Study the drawing (mm; zero at the part's minimum x, y, z) and answer. Round coordinates to 2 decimals unless told otherwise and drop trailing zeros. Loops run counter-clockwise (first coordinate to the right, second up) from the corner with the lowest first, then second, coordinate; pieces in that order, holes last. Notation, with made-up numbers: M -31,20.5 L 9,20.5 A27 cw 9,52.5 Z; hole C 6,46.25 d10. An arc over 180 degrees is marked long. Put each result on its own line as item: value. Start each with the question number.
(1) Straight lines are drawn through the part: line 1 (Z direction, x = 50, y = 5); line 2 (X direction, y = 3.75, z = 120.5). For each, find the intervals that lie inside material, in ascending order.
(2) Section C-C, the plane y = 2 is taken. Determine the outline of the cut face in (x, z).
(3) Section A-A, the plane z = 20 is taken. Determine the outline of the cut face in (x, y), then the cut area to 3 significant figures.
(4) Section D-D, the plane z = 114.5 is taken. Determine the outline of the cut face in (x, y).
(5) Section B-B, the plane x = 50 is taken. Determine the outline of the cut face in (y, z).
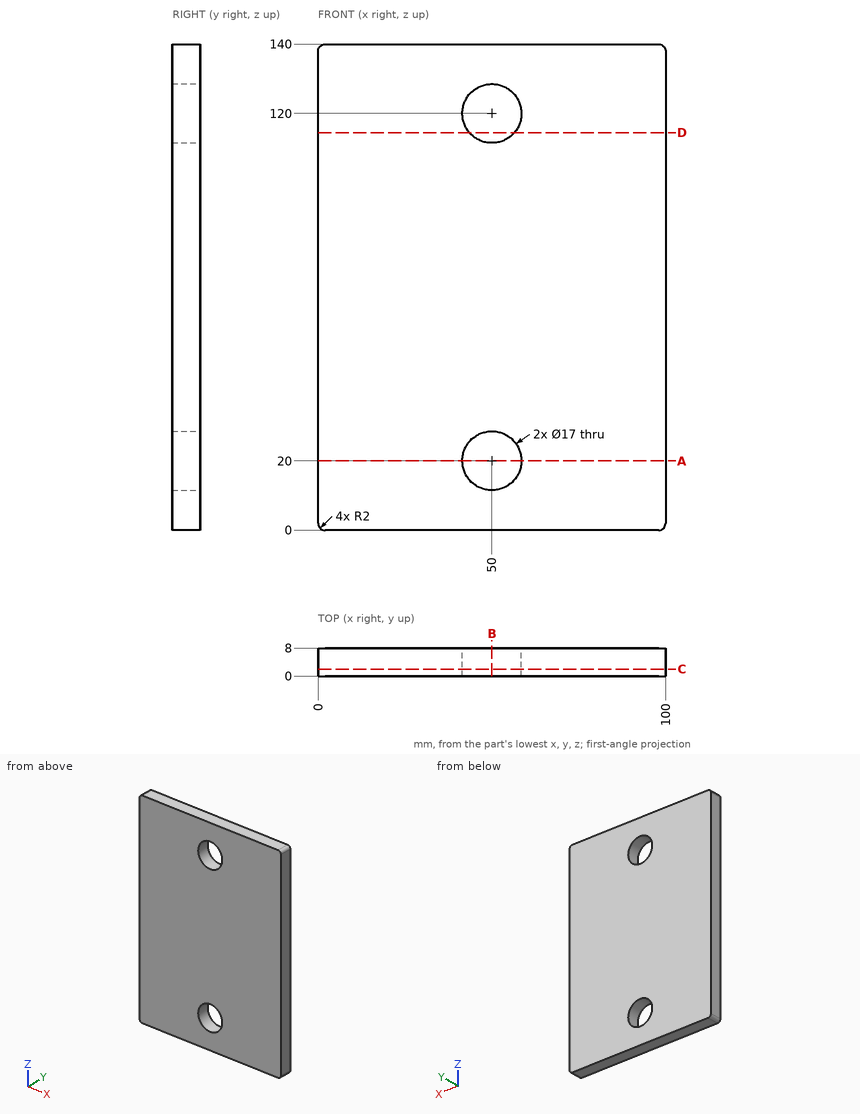
Recorded:
1. line 1: z = 0 to 11.5, 28.5 to 111.5, 128.5 to 140
1. line 2: x = 0 to 41.51, 58.49 to 100
2. outline: M 0,2 A2 ccw 2,0 L 98,0 A2 ccw 100,2 L 100,138 A2 ccw 98,140 L 2,140 A2 ccw 0,138 Z; hole C 50,20 d17; hole C 50,120 d17
3. outline: M 0,0 L 41.5,0 L 41.5,8 L 0,8 Z; M 58.5,0 L 100,0 L 100,8 L 58.5,8 Z
3. area: 664 mm²
4. outline: M 0,0 L 43.52,0 L 43.52,8 L 0,8 Z; M 56.48,0 L 100,0 L 100,8 L 56.48,8 Z
5. outline: M 0,0 L 8,0 L 8,11.5 L 0,11.5 Z; M 0,28.5 L 8,28.5 L 8,111.5 L 0,111.5 Z; M 0,128.5 L 8,128.5 L 8,140 L 0,140 Z
